from build123d import *

# Parameters (mm, degrees)
F0_R     = 13
F1_DEPTH = 120
F2_R     = 5
F4_R     = 13
F5_DEPTH = 22


with BuildPart() as f1:
    # F0 (on Top) → F1 (new body)
    with BuildSketch(Plane.XY):
        Circle(F0_R)
    extrude(amount=F1_DEPTH)

    # F2
    f2_edges = [f1.edges().sort_by_distance(p)[0] for p in [
        (-13, 0, 0),
    ]]
    fillet(f2_edges, radius=F2_R)

    # F4 (on offset) → F5 (join)
    with BuildSketch(Plane.XY.offset(15)):
        Polygon((11.835681, 20.5), (-11.835681, 20.5), (-23.671361, 0), (-11.835681, -20.5), (11.835681, -20.5), (23.671361, 0), align=None)
        Circle(F4_R, mode=Mode.SUBTRACT)
    extrude(amount=F5_DEPTH)


solid = f1.part
Geometry check sheet. Reference: the model listing, model coordinates, mm. A direction names the side the tool comes from. Give positions to 0.01 mm unless a question says otherwise; leave off trailing zeros. Order: outer loops, then holes, each group sorted by start corner. A loop starts at its lowest first (then second) coordinate and runs counter-clockwise, first axis right, second up.
1. Sectioned sample at C-C (y = 17). Record the boundary of the cut face in (x, z).
Completed:
outline: (-13.86, 15) - (13.86, 15) - (13.86, 37) - (-13.86, 37) - close
2. Sectioned sample at D-D (y = -16). Record the boundary of the cut face in (x, z).
Completed:
outline: (-14.43, 15) - (14.43, 15) - (14.43, 37) - (-14.43, 37) - close
3. Depth check by flat-ended pin: pin 1 (4 mm diameter, centred on x = -18.5, z = 29, fed in from -Y); pin 2 (12 mm diameter, centred on x = -13, z = 81, fed in from +Y); pin 3 (5 mm diameter, centred on y = -11, z = 41, fed in from +X). Enter the tip coordinate at first touch or a pass-through.
Completed:
pin 1: stops at y = -12.42
pin 2: stops at y = 10.95
pin 3: stops at x = 9.84
4. Access from +Z, -Z, +X, -X, +Y, -Y to the whole of each face (thin tool, end or side, straight path). Record for faces 1 (the face through (10, 9, 37)), 2 (the face through (-10.316, -7.91, 9.93)), 3 (the face through (17.836, 10.107, 25.846)).
Completed:
face 1: +Z
face 2: -Z
face 3: +Z, -Z, +X, +Y
5. Sectioned sample at A-A (x = 0). Record the boundary of the cut face in (y, z).
Completed:
outline: (-20.5, 15) - (-13, 15) - (-13, 5) arc R5 ccw to (-8, 0) - (8, 0) arc R5 ccw to (13, 5) - (13, 15) - (20.5, 15) - (20.5, 37) - (13, 37) - (13, 120) - (-13, 120) - (-13, 37) - (-20.5, 37) - close
6. Sectioned sample at B-B (z = 39). Record the boundary of the cut face in (x, y), then the cut area to 3 significant figures.
Completed:
outline: circle Ø26 at (0, 0)
area: 531 mm2
7. Scan lines: line 1 (Z direction, x = -9, y = 14); line 2 (Y direction, x = 0.5, z = 110.5); line 3 (X direction, y = -14, z = 31.5). Record each from-to range of solid material in increasing order.
Completed:
line 1: z = 15 to 37
line 2: y = -12.99 to 12.99
line 3: x = -15.59 to 15.59
